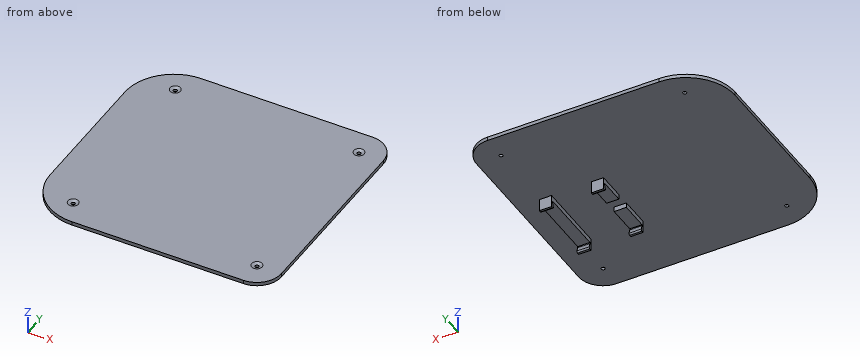
```python
from build123d import *
from OCP.BRepFilletAPI import BRepFilletAPI_MakeChamfer

# Parameters (mm, degrees)
BASE_DEPTH                   = 3
SKETCH2_R                    = 1.5
SCREWHOLES_DEPTH             = 138.963763358
CHAMFER1_SIZE                = 1
CHAMFER1_SIZE2               = 2.747477419
SKETCH3_W                    = 10
SKETCH3_H                    = 55
ARDUINORISERS_DEPTH          = 4
SKETCH4_W                    = 10
SKETCH4_H                    = 1.5
ARDUINOCLAMPSSIDE_DEPTH      = 10
ARDUINOCLAMPSCATCHERS1_DEPTH = 10
ARDUINOCLAMPSCATCHERS2_DEPTH = 10
SKETCH7_W                    = 10
SKETCH7_H                    = 11
ISPSPACE_DEPTH               = 4


with BuildPart() as part:
    # Sketch1 → base (new body)
    with BuildSketch(Plane.XY):
        with BuildLine():
            Line((80, 95), (-60, 95))
            ThreePointArc((-60, 95), (-88.284271247, 83.284271247), (-100, 55))
            Line((-100, 55), (-100, -55))
            ThreePointArc((-100, -55), (-88.284271247, -83.284271247), (-60, -95))
            Line((-60, -95), (80, -95))
            ThreePointArc((80, -95), (94.142135624, -89.142135624), (100, -75))
            Line((100, -75), (100, 75))
            ThreePointArc((100, 75), (94.142135624, 89.142135624), (80, 95))
        make_face()
    extrude(amount=BASE_DEPTH)

    # Sketch2 → screwHoles (cut, through all)
    with BuildSketch(Plane(origin=(0, 0, 0), x_dir=(-1, 0, 0), z_dir=(0, 0, -1))):
        with Locations((-80, 75)):
            Circle(SKETCH2_R)
        with Locations((-80, -75)):
            Circle(SKETCH2_R)
        with Locations((70, -75)):
            Circle(SKETCH2_R)
        with Locations((70, 75)):
            Circle(SKETCH2_R)
    extrude(amount=-SCREWHOLES_DEPTH, mode=Mode.SUBTRACT)

    # Chamfer1: one chamfer whose edges measure the first distance from different faces: ONE call of the kernel's chamfer builder (chamfer() names one face for all edges)
    chamfer1_edges_1 = [part.edges().sort_by_distance(p)[0] for p in [
        (81.5, 75, 3),
    ]]
    chamfer1_side_1 = [part.faces().sort_by_distance(p)[0] for p in [
        (81.5, 75, 1.5),
    ]]
    chamfer1_edges_2 = [part.edges().sort_by_distance(p)[0] for p in [
        (81.5, -75, 3),
    ]]
    chamfer1_side_2 = [part.faces().sort_by_distance(p)[0] for p in [
        (81.5, -75, 1.5),
    ]]
    chamfer1_edges_3 = [part.edges().sort_by_distance(p)[0] for p in [
        (-68.5, -75, 3),
    ]]
    chamfer1_side_3 = [part.faces().sort_by_distance(p)[0] for p in [
        (-68.5, -75, 1.5),
    ]]
    chamfer1_edges_4 = [part.edges().sort_by_distance(p)[0] for p in [
        (-68.5, 75, 3),
    ]]
    chamfer1_side_4 = [part.faces().sort_by_distance(p)[0] for p in [
        (-68.5, 75, 1.5),
    ]]
    chamfer1 = BRepFilletAPI_MakeChamfer(part.part.solid().wrapped)
    for e in chamfer1_edges_1:
        chamfer1.Add(CHAMFER1_SIZE, CHAMFER1_SIZE2, e.wrapped, chamfer1_side_1[0].wrapped)  # the first distance lies on this face
    for e in chamfer1_edges_2:
        chamfer1.Add(CHAMFER1_SIZE, CHAMFER1_SIZE2, e.wrapped, chamfer1_side_2[0].wrapped)  # the first distance lies on this face
    for e in chamfer1_edges_3:
        chamfer1.Add(CHAMFER1_SIZE, CHAMFER1_SIZE2, e.wrapped, chamfer1_side_3[0].wrapped)  # the first distance lies on this face
    for e in chamfer1_edges_4:
        chamfer1.Add(CHAMFER1_SIZE, CHAMFER1_SIZE2, e.wrapped, chamfer1_side_4[0].wrapped)  # the first distance lies on this face
    add(Compound.cast(chamfer1.Shape()), mode=Mode.REPLACE)

    # Sketch3 → arduinoRisers (add)
    with BuildSketch(Plane(origin=(0, 0, 0), x_dir=(-1, 0, 0), z_dir=(0, 0, -1))):
        with Locations((-76, -12)):
            Rectangle(SKETCH3_W, SKETCH3_H)
        with Locations((-33.5, -12)):
            Rectangle(SKETCH3_W, SKETCH3_H)
    extrude(amount=ARDUINORISERS_DEPTH)

    # Sketch4 → arduinoClampsSide (add)
    with BuildSketch(Plane(origin=(0, 0, 0), x_dir=(-1, 0, 0), z_dir=(0, 0, -1))):
        with Locations((-76, -40.25)):
            Rectangle(SKETCH4_W, SKETCH4_H)
        with Locations((-33.5, -40.25)):
            Rectangle(SKETCH4_W, SKETCH4_H)
        with Locations((-76, 16.25)):
            Rectangle(SKETCH4_W, SKETCH4_H)
        with Locations((-33.5, 16.25)):
            Rectangle(SKETCH4_W, SKETCH4_H)
    extrude(amount=ARDUINOCLAMPSSIDE_DEPTH)

    # Sketch5 → arduinoClampsCatchers1 (add)
    with BuildSketch(Plane(origin=(81, 0, 0), x_dir=(0, 0, -1), z_dir=(1, 0, 0))):
        with BuildLine():
            Line((5, 15.5), (8.712652114, 14.386204366))
            ThreePointArc((8.712652114, 14.386204366), (9.59693053, 14.541737723), (10, 15.344030651))
            Line((10, 15.344030651), (10, 15.5))
            Line((10, 15.5), (5, 15.5))
        make_face()
        with BuildLine():
            Line((5, -39.5), (8.712652114, -38.386204366))
            ThreePointArc((8.712652114, -38.386204366), (9.59693053, -38.541737723), (10, -39.344030651))
            Line((10, -39.344030651), (10, -39.5))
            Line((10, -39.5), (5, -39.5))
        make_face()
    extrude(amount=-ARDUINOCLAMPSCATCHERS1_DEPTH)

    # Sketch6 → arduinoClampsCatchers2 (add)
    with BuildSketch(Plane(origin=(38.5, 0, 0), x_dir=(0, 0, -1), z_dir=(1, 0, 0))):
        with BuildLine():
            Line((5, 15.5), (8.712652114, 14.386204366))
            ThreePointArc((8.712652114, 14.386204366), (9.59693053, 14.541737723), (10, 15.344030651))
            Line((10, 15.344030651), (10, 15.5))
            Line((10, 15.5), (5, 15.5))
        make_face()
        with BuildLine():
            Line((8.712652114, -38.386204366), (5, -39.5))
            Line((5, -39.5), (10, -39.5))
            Line((10, -39.5), (10, -39.344030651))
            ThreePointArc((10, -39.344030651), (9.59693053, -38.541737723), (8.712652114, -38.386204366))
        make_face()
    extrude(amount=-ARDUINOCLAMPSCATCHERS2_DEPTH)

    # Sketch7 → ISPspace (cut)
    with BuildSketch(Plane(origin=(0, 0, -4), x_dir=(-1, 0, 0), z_dir=(0, 0, -1))):
        with Locations((-33.5, -11)):
            Rectangle(SKETCH7_W, SKETCH7_H)
    extrude(amount=-ISPSPACE_DEPTH, mode=Mode.SUBTRACT)


solid = part.part
```
CAD build for the part. Positions are in the model's coordinates, mm. Round coordinates to 2 decimals unless told otherwise and drop trailing zeros. Loops run counter-clockwise (first coordinate to the right, second up) from the corner with the lowest first, then second, coordinate; pieces in that order, holes last. Notation, with made-up numbers: M 41.25,27 L 46.25,27 A34 cw 46.25,59 Z; hole C 19,-16 d10. An arc over 180 degrees is marked long. Use a Markdown table: item, result. Add a question column.
(1) Flat gauge pins, fed straight in: pin 1 (4 mm diameter, centred on y = 32, z = -0.5, fed in from +X); pin 2 (5 mm diameter, centred on x = -1.5, y = 19.5, fed in from -Z); pin 3 (3 mm diameter, centred on y = -28.5, z = -3.5, fed in from +X); pin 4 (1.1 mm diameter, centred on x = 31, z = -4.5, fed in from +Y). Where does each tip first touch, or does it go through?
(2) Cut at C-C (x = -40.5). Give the cut face in (y, z), and give its area (3 significant figures).
(3) Cut at D-D (y = -49). Give the cut face in (x, z), and give its area (3 significant figures).
(4) Cut at A-A (z = -2). Give the cut face in (x, y), and give its area (3 significant figures).
(5) Cut at B-B (y = -20.5). Give the cut face in (x, z), and give its area (3 significant figures).
(6) Drill centre lines: line 1 (Y direction, x = 80, z = 0.65); line 2 (X direction, y = -75, z = 0.65); line 3 (Y direction, x = -70, z = 1.3). Where is each one in solid material? Low to high.
Geometry says:
| question | item | result |
|---|---|---|
| 1 | pin 1 | stops at x = 100 |
| 1 | pin 2 | stops at z = 0 |
| 1 | pin 3 | stops at x = 81 |
| 1 | pin 4 | stops at y = 17 |
| 2 | outline | M -95,0 L 95,0 L 95,3 L -95,3 Z |
| 2 | area | 570 mm² |
| 3 | outline | M -100,0 L 100,0 L 100,3 L -100,3 Z |
| 3 | area | 600 mm² |
| 4 | outline | M 28.5,-41 L 38.5,-41 L 38.5,-16.5 L 28.5,-16.5 Z; M 28.5,-5.5 L 38.5,-5.5 L 38.5,17 L 28.5,17 Z; M 71,-41 L 81,-41 L 81,17 L 71,17 Z |
| 4 | area | 1,050 mm² |
| 5 | outline | M -100,0 L 28.5,0 L 28.5,-4 L 38.5,-4 L 38.5,0 L 71,0 L 71,-4 L 81,-4 L 81,0 L 100,0 L 100,3 L -100,3 Z |
| 5 | area | 680 mm² |
| 6 | line 1 | y = -95 to -76.5, -73.5 to 73.5, 76.5 to 95 |
| 6 | line 2 | x = -94.64 to -71.5, -68.5 to 78.5, 81.5 to 100 |
| 6 | line 3 | y = -93.73 to -76.5, -73.5 to 73.5, 76.5 to 93.73 |
